Input: part model. Units: mm. Frame: model coordinates. Face numbers are marked on the shaded views. A direction names the side the tool comes from. Round coordinates to 2 decimals unless told otherwise and drop trailing zeros. Loops run counter-clockwise (first coordinate to the right, second up) from the corner with the lowest first, then second, coordinate; pieces in that order, holes last. Notation, with made-up numbers: (82.5, 81) -> (114.5, 81) arc R20 cw to (114.5, 120) -> close; hole circle Ø10 at (-17, 40). An arc over 180 degrees is marked (long way). Answer as a JSON object with one key per item and string values.
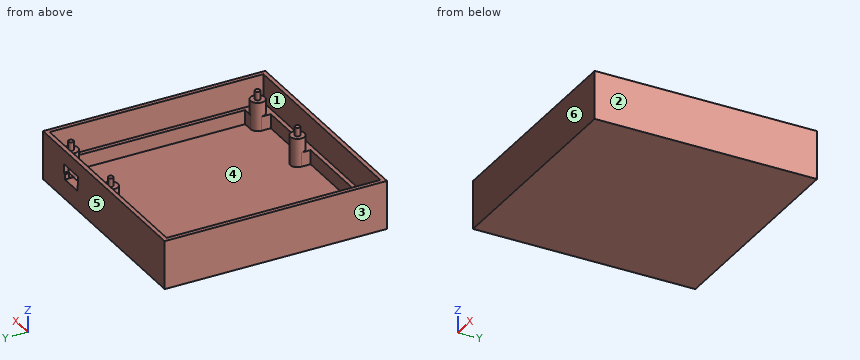
Autodesk Inventor part; units mm, degrees
ref_plane "YZ Plane" through (0, 0, 0) normal (1, 0, 0) x (0, 1, 0)
ref_plane "XZ Plane" through (0, 0, 0) normal (0, 1, 0) x (-1, 0, 0)
ref_plane "XY Plane" through (0, 0, 0) normal (0, 0, 1) x (1, 0, 0)
sketch "USB_Micro" plane through (0, 0, 0) normal (0, 0, 1) x (1, 0, 0)
  line L0 (-6.7, 3.4) -> (-6.7, 2.0438)
  line L1 (-7.2, 1.6938) -> (-6.7, 2.0438)
  line L2 (-7.2, 1.6938) -> (-7.2, 0.3)
  line L3 (-7.2, 0.3) -> (-0.3, 0.3)
  line L4 (-0.3, 0.3) -> (-0.3, 1.6938)
  line L5 (-0.8, 2.0438) -> (-0.3, 1.6938)
  line L6 (-6.7, 3.4) -> (-0.8, 3.4)
  line L7 (-0.8, 3.4) -> (-0.8, 2.0438)
  line L8 (-0.8, 0.8) -> (-6.7, 0.8)
  line L9 (-6.7, 0.8) -> (-6.7, 1.4335)
  line L10 (-6.7, 1.4335) -> (-6.2, 1.7835)
  line L11 (-6.2, 1.7835) -> (-6.2, 2.9)
  line L12 (-6.2, 2.9) -> (-1.3, 2.9)
  line L13 (-1.3, 2.9) -> (-1.3, 1.7835)
  line L14 (-1.3, 1.7835) -> (-0.8, 1.4335)
  line L15 (-0.8, 1.4335) -> (-0.8, 0.8)
  point P0 (-3.75, 0.3)
  dimension "d42" = 0.5
sketch "Skizze1" plane through (0, 0, 0) normal (0, 0, 1) x (1, 0, 0)
  line L0 (-39, -39) -> (39, -39)
  line L1 (39, -39) -> (39, 39)
  line L2 (39, 39) -> (-39, 39)
  line L3 (-39, 39) -> (-39, -39)
  line L4 (-39, -39) -> (39, 39) construction
  line L5 (39, -39) -> (-39, 39) construction
  line L6 (-37.5, -37.5) -> (37.5, -37.5)
  line L7 (37.5, -37.5) -> (37.5, 37.5)
  line L8 (37.5, 37.5) -> (-37.5, 37.5)
  line L9 (-37.5, 37.5) -> (-37.5, -37.5)
  line L10 (-37.5, -37.5) -> (37.5, 37.5) construction
  line L11 (37.5, -37.5) -> (-37.5, 37.5) construction
  line L12 (-37.5, 37.5) -> (-36, 37.5)
  line L13 (-36, 37.5) -> (-36, -37.5)
  line L14 (-36, -37.5) -> (-37.5, -37.5)
  line L15 (-37.5, -37.5) -> (-37.5, 37.5)
  line L16 (36, 37.5) -> (37.5, 37.5)
  line L17 (37.5, 37.5) -> (37.5, -37.5)
  line L18 (37.5, -37.5) -> (36, -37.5)
  line L19 (36, -37.5) -> (36, 37.5)
  line L20 (-36, -36) -> (36, -36)
  line L21 (36, -36) -> (36, -37.5)
  line L22 (36, -37.5) -> (-36, -37.5)
  line L23 (-36, -37.5) -> (-36, -36)
  line L24 (36, 37.5) -> (-36, 37.5)
  line L25 (-36, 37.5) -> (-36, 36)
  line L26 (-36, 36) -> (36, 36)
  line L27 (36, 36) -> (36, 37.5)
  point P0 (0, 0)
  dimension "d0" = 78
  dimension "d1" = 78
  dimension "d2" = 75
  dimension "d3" = 75
  dimension "d46" = 1.5
  dimension "d47" = 1.5
  dimension "d48" = 1.5
  dimension "d52" = 1.5
extrude "Extrusion1" add sketch "Skizze1" along normal blind 15
extrude "Extrusion9" add sketch "Skizze1" along normal blind 5 contours L9 L8 L13 L6 | L13 L20 L19 L6 | L19 L8 L7 L6 | L8 L19 L26 L13
extrude "Extrusion6" add sketch "Skizze1" against normal blind 2 contours L3 L2 L1 L0 | L9 L8 L13 L6 | L13 L20 L19 L6 | L19 L8 L7 L6 | L13 L26 L19 L20 | L8 L19 L26 L13
sketch "Skizze5" plane through (0, 0, 0) normal (0, 0, 1) x (1, 0, 0)
  circle A0 centre (32.5, -32.75) radius 0.9
  circle A1 centre (32.5, 32.75) radius 0.9
  circle A2 centre (7, -32.75) radius 0.9
  circle A3 centre (7, 32.75) radius 0.9
  circle A4 centre (32.5, 32.75) radius 2.5
  circle A5 centre (7, 32.75) radius 2.5
  circle A6 centre (32.5, -32.75) radius 2.5
  circle A7 centre (7, -32.75) radius 2.5
  line L0 (-54.6, 0) -> (54.6, 0)
  line L1 (0, -54.6) -> (0, 54.6)
  line L2 (36, 36) -> (36, -36)
  line L3 (-36, 36) -> (36, 36)
  line L4 (36, -36) -> (-36, -36)
  line L5 (9.5, 32.75) -> (9.5, 36)
  line L6 (4.5, 32.75) -> (4.5, 36)
  line L7 (4.5, 36) -> (9.5, 36)
  line L8 (30, 32.75) -> (30, 36)
  line L9 (30, 36) -> (36, 36)
  line L10 (32.5, 30.25) -> (36, 30.25)
  line L11 (36, 30.25) -> (36, 36)
  line L12 (32.5, -30.25) -> (36, -30.25)
  line L13 (36, -30.25) -> (36, -36)
  line L14 (30, -32.75) -> (30, -36)
  line L15 (30, -36) -> (36, -36)
  line L16 (9.5, -32.75) -> (9.5, -36)
  line L17 (4.5, -32.75) -> (4.5, -36)
  line L18 (4.5, -36) -> (9.5, -36)
  point P0 (0, 0)
  dimension "d28" = 1.8
  dimension "d33" = 5
  dimension "d34" = 65.5
  dimension "d35" = 25.5
  dimension "d36" = 32.5
  dimension "d37" = 32.75
  dimension "d51" = 32.75
extrude "Extrusion7" add sketch "Skizze5" along normal blind 10 contours A4 | A5 | A6 | A7
sketch "Skizze6" plane through (-39, 39, 15) normal (0, 1, 0) x (1, 0, 0)
  line L0 (63.71, 5.7) -> (56.21, 5.7)
  line L1 (63.71, 7.55) -> (63.71, 5.7)
  line L2 (63.71, 7.55) -> (63.21, 7.9)
  line L3 (63.21, 7.9) -> (63.21, 9.4)
  line L4 (56.71, 9.4) -> (63.21, 9.4)
  line L5 (56.71, 7.9) -> (56.71, 9.4)
  line L6 (56.21, 7.55) -> (56.71, 7.9)
  line L7 (56.21, 7.55) -> (56.21, 5.7)
  line L8 (56.51, 6) -> (63.41, 6)
  line L9 (56.51, 7.3938) -> (56.51, 6)
  line L10 (57.01, 7.7438) -> (56.51, 7.3938)
  line L11 (57.01, 9.1) -> (57.01, 7.7438)
  line L12 (62.91, 9.1) -> (57.01, 9.1)
  line L13 (62.91, 9.1) -> (62.91, 7.7438)
  line L14 (62.91, 7.7438) -> (63.41, 7.3938)
  line L15 (63.41, 7.3938) -> (63.41, 6)
  line L16 (64.46, 4.95) -> (55.46, 4.95)
  line L17 (55.46, 4.95) -> (55.46, 7.9405)
  line L18 (55.46, 7.9405) -> (55.96, 8.2905)
  line L19 (55.96, 8.2905) -> (55.96, 10.15)
  line L20 (55.96, 10.15) -> (63.96, 10.15)
  line L21 (63.96, 10.15) -> (63.96, 8.2905)
  line L22 (63.96, 8.2905) -> (64.46, 7.9405)
  line L23 (64.46, 7.9405) -> (64.46, 4.95)
  point P0 (39, 15)
  dimension "d45" = 0.75
extrude "Extrusion8" cut sketch "Skizze6" against normal up to surface (3 mm away) contours L0 L7 L6 L5 L4 L3 L2 L1 | L9 L10 L11 L12 L13 L14 L15 L8 | L16 L17 L18 L19 L20 L21 L22 L23
extrude "Extrusion10" add sketch "Skizze5" along normal blind 13 contours A0 | A1 | A2 | A3
extrude "Extrusion11" add sketch "Skizze5" along normal up to surface (5 mm away) contours A4 L8 L3 L2 L10 | L5 A5 L6 L3 | L2 L4 L14 A6 L12 | L17 A7 L16 L4
equation "\"d0\" = d1"
equation "\"d2\" = d3"
equation "\"d47\" = d46"
equation "\"d48\" = d46"
equation "\"d52\" = d46"
properties part number "Sensorlamp_Base"
1) Section A-A, the plane x = -10.5. Output: boundary loops of the cut face in (y, z).
Output:
{"outline": "(-39, -2) -> (39, -2) -> (39, 15) -> (37.5, 15) -> (37.5, 5) -> (36, 5) -> (36, 0) -> (-36, 0) -> (-36, 5) -> (-37.5, 5) -> (-37.5, 15) -> (-39, 15) -> close"}
2) Section B-B, the plane z = 14. Output: boundary loops of the cut face in (x, y), plus the area to 3 significant figures.
Output:
{"outline": "(-39, -39) -> (39, -39) -> (39, 39) -> (-39, 39) -> close; hole (-37.5, -37.5) -> (37.5, -37.5) -> (37.5, 37.5) -> (-37.5, 37.5) -> close", "area": "459 mm^2"}
3) Contact query for flat-ended pins moving along their axis: P1, Ø5, axis at x = -8, y = 30, coming from the +Z side; P2, Ø5.5, axis at x = 6.5, y = -32, coming from the +Z side. Output: stop coordinate, or through.
Output:
{"P1": "stops at z = 0", "P2": "stops at z = 13"}
4) Reachability of the marked faces 1 and 2 from +Z, -Z, +X, -X, +Y, -Y: full face, straight path, thin tool, end or side. Return the list, or none.
Output:
{"face 1": "+Z", "face 2": "+Z, -Z, +X, +Y, -Y"}
5) Draft query along Y for the marked faces 3, 4, 5 and 6. Return one class per face: +Y half, -Y half, draft (parallel to the pull), parting line (faces both ways), or undercut.
Output:
{"face 3": "draft", "face 4": "undercut", "face 5": "+Y half", "face 6": "-Y half"}
6) Section D-D, the plane z = 1.5. Output: boundary loops of the cut face in (x, y).
Output:
{"outline": "(-39, -39) -> (39, -39) -> (39, 39) -> (-39, 39) -> close; hole (-36, -36) -> (4.5, -36) -> (4.5, -32.75) arc R2.5 cw to (9.5, -32.75) -> (9.5, -36) -> (30, -36) -> (30, -32.75) arc R2.5 cw to (32.5, -30.25) -> (36, -30.25) -> (36, 30.25) -> (32.5, 30.25) arc R2.5 cw to (30, 32.75) -> (30, 36) -> (9.5, 36) -> (9.5, 32.75) arc R2.5 cw to (4.5, 32.75) -> (4.5, 36) -> (-36, 36) -> close"}
7) Ray query, probe 1 along Y at (x, z) = (16, 9.75); probe 2 along Y at (x, z) = (22.5, 0.25). Return the intervals inside material, ascending.
Output:
{"probe 1": "y = -39 to -37.5, 37.5 to 39", "probe 2": "y = -39 to -36, 36 to 39"}
